from build123d import *

# Parameters (mm, degrees)
SKETCH1_W                      = 11.5
SKETCH1_H                      = 33
BOSS_EXTRUDE1_DEPTH            = 12.65
FILLET1_R                      = 3
CUT_EXTRUDE1_REACH             = 25.76
CBORE_FOR_M4_SHCS1_D           = 4.3
CBORE_FOR_M4_SHCS1_CBORE_D     = 8
CBORE_FOR_M4_SHCS1_CBORE_DEPTH = 4


with BuildPart() as part:
    # Sketch1 → Boss-Extrude1 (new body)
    with BuildSketch(Plane.XY):
        Rectangle(SKETCH1_W, SKETCH1_H)
    extrude(amount=BOSS_EXTRUDE1_DEPTH)

    # Fillet1
    fillet1_edges = [part.edges().sort_by_distance(p)[0] for p in [
        (5.75, -16.5, 6.325),
        (-5.75, -16.5, 6.325),
        (-5.75, 16.5, 6.325),
        (5.75, 16.5, 6.325),
    ]]
    fillet(fillet1_edges, radius=FILLET1_R)

    # Sketch2 → Cut-Extrude1 (cut, up to next)
    with BuildSketch(Plane(origin=(5.75, 0, 0), x_dir=(0, 0, -1), z_dir=(1, 0, 0)), mode=Mode.PRIVATE) as cut_extrude1_sk1:
        with BuildLine():
            Line((-12.65, 8), (-12.65, -8))
            ThreePointArc((-12.65, -8), (-4.65, 0), (-12.65, 8))
        make_face()
    cut_extrude1_tool1 = extrude(cut_extrude1_sk1.sketch, amount=-CUT_EXTRUDE1_REACH, mode=Mode.PRIVATE) & part.part
    add(cut_extrude1_tool1.solids().sort_by_distance((5.75, 0, 9.254695))[0], mode=Mode.SUBTRACT)

    # CBORE for M4 SHCS1 (through all)
    with Locations(Plane(origin=(0, 0, 0), x_dir=(-1, 0, 0), z_dir=(0, 0, -1))):
        with Locations((0, 11.5), (0, -11.5)):
            CounterBoreHole(CBORE_FOR_M4_SHCS1_D / 2, CBORE_FOR_M4_SHCS1_CBORE_D / 2, CBORE_FOR_M4_SHCS1_CBORE_DEPTH)


solid = part.part
Geometry: final body of the model. Coordinates: model frame, mm. A direction names the side the tool comes from. Coordinates: 2 decimals unless noted, no trailing zeros. Order: outer loops, then holes, each group sorted by start corner. A loop starts at its lowest first (then second) coordinate and runs counter-clockwise, first axis right, second up.
(1) Draft query along Y for faces 1 (the face through (-2.15, -11.41, 8.39)), 2 (the face through (4.89, 15.6, 6.41)), 3 (the face through (-1.706, 10.192, 8.386)), 4 (the face through (4.85, -15.64, 6.41)). Return one class per face: pulls with the +Y half, pulls with the -Y half, needs draft (parallel to the pull), parting line crosses it, or undercut.
(2) Section query D-D (z = 8.25). Return the cut outline in (x, y).
(3) Material intervals for probe 1 along Y at (x, z) = (0, 2.4); probe 2 along Y at (x, z) = (1, 4.25); probe 3 along Y at (x, z) = (0, 8), sorted ascending.
(4) Section query A-A (x = 0). Return the cut outline in (y, z).
(5) First-contact query: pin 1 (6 mm diameter, centred on x = 4.5, y = -7, fed in from -Z); pin 2 (1.5 mm diameter, centred on x = -3, y = 0.5, fed in from +Z); pin 3 (2.5 mm diameter, centred on x = -1, y = -10, fed in from -Z); pin 4 (1 mm diameter, centred on x = -4, y = 1.5, fed in from +Z). Flat tips, straight axial feed; report the tip coordinate or a pass-through.
(6) Section query C-C (z = 5.5). Return the cut outline in (x, y).
(7) Access query for faces 5 (the face through (5.75, 0, 3)), 6 (the face through (-2, -13, 4)). Directions: +Z, -Z, +X, -X, +Y, -Y. A direction counts if a zero-diameter tool reaches every point of the face in a straight line with its end or side. Return the directions, or none.
(8) Section query B-B (y = 11.5). Return the cut outline in (x, z), plus the area to 3 significant figures.
Solution:
1. face 1: undercut
1. face 2: pulls with the +Y half
1. face 3: undercut
1. face 4: pulls with the -Y half
2. outline: (-5.75, -13.5) arc R3 ccw to (-2.75, -16.5) - (2.75, -16.5) arc R3 ccw to (5.75, -13.5) - (5.75, -6.68) - (-5.75, -6.68) - close; (-5.75, 6.68) - (5.75, 6.68) - (5.75, 13.5) arc R3 ccw to (2.75, 16.5) - (-2.75, 16.5) arc R3 ccw to (-5.75, 13.5) - close; hole circle Ø4.3 at (0, -11.5); hole circle Ø4.3 at (0, 11.5)
3. probe 1: y = -16.5 to -15.5, -7.5 to 7.5, 15.5 to 16.5
3. probe 2: y = -16.5 to -13.4, -9.6 to 9.6, 13.4 to 16.5
3. probe 3: y = -16.5 to -13.65, -9.35 to -6.51, 6.51 to 9.35, 13.65 to 16.5
4. outline: (-16.5, 0) - (-15.5, 0) - (-15.5, 4) - (-13.65, 4) - (-13.65, 12.65) - (-16.5, 12.65) - close; (-9.35, 4) - (-7.5, 4) - (-7.5, 0) - (7.5, 0) - (7.5, 4) - (9.35, 4) - (9.35, 12.65) - (8, 12.65) arc R8 cw to (-8, 12.65) - (-9.35, 12.65) - close; (13.65, 4) - (15.5, 4) - (15.5, 0) - (16.5, 0) - (16.5, 12.65) - (13.65, 12.65) - close
5. pin 1: stops at z = 0
5. pin 2: stops at z = 4.75
5. pin 3: stops at z = 4
5. pin 4: stops at z = 4.9
6. outline: (-5.75, -13.5) arc R3 ccw to (-2.75, -16.5) - (2.75, -16.5) arc R3 ccw to (5.75, -13.5) - (5.75, -3.59) - (-5.75, -3.59) - close; (-5.75, 3.59) - (5.75, 3.59) - (5.75, 13.5) arc R3 ccw to (2.75, 16.5) - (-2.75, 16.5) arc R3 ccw to (-5.75, 13.5) - close; hole circle Ø4.3 at (0, -11.5); hole circle Ø4.3 at (0, 11.5)
7. face 5: +Z, -Z, +X, +Y, -Y
7. face 6: -Z
8. outline: (-5.75, 0) - (-4, 0) - (-4, 4) - (-2.15, 4) - (-2.15, 12.65) - (-5.75, 12.65) - close; (2.15, 4) - (4, 4) - (4, 0) - (5.75, 0) - (5.75, 12.65) - (2.15, 12.65) - close
8. area: 76.3 mm2
